CAD build for the part. Positions are in the model's coordinates, mm. A direction names the side the tool comes from. Coordinates: 2 decimals unless noted, no trailing zeros. Loops run counter-clockwise (first coordinate to the right, second up) from the corner with the lowest first, then second, coordinate; pieces in that order, holes last. Notation, with made-up numbers: (37, 2.25) -> (48, 2.25) arc R20 ccw to (48, 37.25) -> close; hole circle Ø5 at (24.25, 21.25). An arc over 180 degrees is marked (long way). Write each question's results on one line, items separated by ' | '.
Autodesk Inventor part; units mm, degrees
ref_plane "YZ Plane" through (0, 0, 0) normal (1, 0, 0) x (0, 1, 0)
ref_plane "XZ Plane" through (0, 0, 0) normal (0, 1, 0) x (-1, 0, 0)
ref_plane "XY Plane" through (0, 0, 0) normal (0, 0, 1) x (1, 0, 0)
sketch "Sketch1" plane through (0, 0, 0) normal (1, 0, 0) x (0, 1, 0)
  line L0 (45, 0) -> (0, 0)
  circle A0 centre (130, 235) radius 11
  line L1 (73.2002, 0) -> (73.2002, 46.6199)
  line L2 (77.2194, 61.6199) -> (155.9808, 198.0385)
  line L3 (160, 213.0385) -> (160, 235)
  arc A1 (160, 235) -> (130, 265) centre (130, 235) ccw
  line L4 (130, 235) -> (130, 265) construction
  line L5 (130, 235) -> (160, 235) construction
  line L6 (130, 265) -> (-45, 265)
  circle A2 centre (-45, 0) radius 18
  line L7 (0, 0) -> (0, 265)
  circle A3 centre (-45, 235) radius 13
  arc A4 (-45, 265) -> (-75, 235) centre (-45, 235) ccw
  line L8 (-45, 235) -> (-75, 235) construction
  line L9 (-45, 235) -> (-45, 265) construction
  line L10 (-75, 235) -> (-75, 39.1421)
  line L11 (0, 0) -> (-45, 0)
  circle A5 centre (130, -235) radius 11
  line L12 (73.2002, 0) -> (73.2002, -46.6199)
  line L13 (77.2194, -61.6199) -> (155.9808, -198.0385)
  line L14 (160, -213.0385) -> (160, -235)
  arc A6 (130, -265) -> (160, -235) centre (130, -235) ccw
  line L15 (130, -265) -> (-45, -265)
  circle A7 centre (-45, -235) radius 13
  arc A8 (-75, -235) -> (-45, -265) centre (-45, -235) ccw
  line L16 (-45, -235) -> (-75, -235) construction
  line L17 (-75, -235) -> (-75, -39.1421)
  arc A9 (155.9808, 198.0385) -> (160, 213.0385) centre (130, 213.0385) ccw
  arc A10 (77.2194, 61.6199) -> (73.2002, 46.6199) centre (103.2002, 46.6199) ccw
  arc A11 (73.2002, -46.6199) -> (77.2194, -61.6199) centre (103.2002, -46.6199) ccw
  arc A12 (160, -213.0385) -> (155.9808, -198.0385) centre (130, -213.0385) ccw
  line L18 (-77.9289, 32.0711) -> (-82.0711, 27.9289)
  line L19 (-85, 20.8579) -> (-85, 0)
  line L20 (-77.9289, -32.0711) -> (-82.0711, -27.9289)
  line L21 (-85, -20.8579) -> (-85, 0)
  arc A13 (-77.9289, 32.0711) -> (-75, 39.1421) centre (-85, 39.1421) ccw
  arc A14 (-82.0711, 27.9289) -> (-85, 20.8579) centre (-75, 20.8579) ccw
  arc A15 (-85, -20.8579) -> (-82.0711, -27.9289) centre (-75, -20.8579) ccw
  arc A16 (-75, -39.1421) -> (-77.9289, -32.0711) centre (-85, -39.1421) ccw
  point P0 (73.2002, 54.6584)
  point P1 (160, 205)
  point P2 (-75, -35)
  point P3 (48.2002, -10.5242)
  point P4 (73.2002, -54.6584)
  point P5 (160, -205)
  point P6 (-85, 25)
  point P7 (-75, 35)
  point P8 (-85, -25)
  dimension "d1" = 22
  dimension "d2" = 470
  dimension "d3" = 90
  dimension "d4" = 36
  dimension "d7" = 30
  dimension "d8" = 26
  dimension "d9" = 90
  dimension "d11" = 25
  dimension "d12" = 85
  dimension "d13" = 90
  dimension "d14" = 30
  dimension "d15" = 30
  dimension "d16" = 30
  dimension "d19" = 45
  dimension "d20" = 40
  dimension "d21" = 50
  dimension "d22" = 10
extrude "Extrusion1" add sketch "Sketch1" along normal mid plane 25.4
properties part number "Balancim_Duplicador"
Q1. Cut at C-C on z = 82.5. Write the cut outline in (x, y), and give its area (3 significant figures).
Results are:
outline: (-12.7, -75) -> (12.7, -75) -> (12.7, 89.27) -> (-12.7, 89.27) -> close | area: 4,170 mm^2
Q2. Cut at A-A on z = 0. Write the cut outline in (x, y).
Results are:
outline: (-12.7, -85) -> (12.7, -85) -> (12.7, -63) -> (-12.7, -63) -> close; (-12.7, -27) -> (12.7, -27) -> (12.7, 73.2) -> (-12.7, 73.2) -> close
Q3. Cut at D-D on z = -80. Write the cut outline in (x, y), and give its area (3 significant figures).
Results are:
outline: (-12.7, -75) -> (12.7, -75) -> (12.7, 87.83) -> (-12.7, 87.83) -> close | area: 4,140 mm^2
Q4. Pull direction Y, two halves, no side cores. Call faces 4 (the cylindrical face through (-0.178, 151.445, -255.979)), 5 (the flat face through (0, -85, 0)), 6 (the flat face through (0, 44, -265)), 7 (the cylindrical face through (-0.18, -46.69, -247.89)): +Y half, -Y half, draft (parallel to the pull), parting line (faces both ways), or undercut.
Results are:
face 4: +Y half | face 5: -Y half | face 6: draft | face 7: undercut
Q5. Cut at B-B on x = -7.75. Give the number of separate pieces and of enclosed holes in the cut face, and give its area (3 significant figures).
Results are:
separate pieces: 1 | enclosed holes: 5 | area: 99,000 mm^2
Q6. Which spindle directions (+Z, -Z, +X, -X, +Y, -Y) get a long thin tool onto all of the face, cutting with end or side? Do faces 1 (the flat face through (0, -75, 138)), 2 (the flat face through (0, -75, -138)), 3 (the flat face through (-0.178, 116.049, 128.874)). Say none if no direction does.
Results are:
face 1: +Z, +X, -X, -Y | face 2: -Z, +X, -X, -Y | face 3: +X, -X, +Y
Q7. Wall check: L1, parallel to Z at x = -6.5, y = -45; L2, parallel to Z at x = -7, y = 130; L3, parallel to Y at x = -9.25, z = 39. Give the ranges that are in metal, low to high. Write a range as from..to.
Results are:
L1: -265..-248, -222..-18, 18..222, 248..265 | L2: -265..-246, -224..-153.04, 153.04..224, 246..265 | L3: -75..73.2
Q8. Drop flat-ended pins along their axis: pin 1 (17.5 mm diameter, centred on y = 130, z = -235, fed in from -X); pin 2 (1 mm diameter, centred on x = 6.5, z = -103, fed in from -Y); pin 3 (7.5 mm diameter, centred on x = -3, z = -17.5, fed in from +Y); pin 4 (1 mm diameter, centred on x = -4.5, y = -60, fed in from -Z). Give the stop position or say it passes through.
Results are:
pin 1: through | pin 2: y = -75 | pin 3: y = 73.2 | pin 4: z = -261.26
